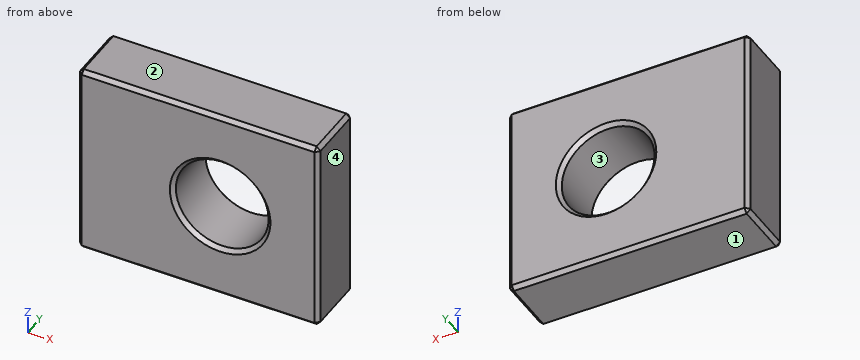
Autodesk Inventor part; units mm, degrees
ref_plane "YZ Plane" through (0, 0, 0) normal (1, 0, 0) x (0, 1, 0)
ref_plane "XZ Plane" through (0, 0, 0) normal (0, 1, 0) x (-1, 0, 0)
ref_plane "XY Plane" through (0, 0, 0) normal (0, 0, 1) x (1, 0, 0)
sketch "Sketch1" plane through (0, 0, 0) normal (0, 1, 0) x (-1, 0, 0)
  line L0 (0, 0) -> (-15.85, 0) construction
  line L1 (-15.85, 0) -> (-15.85, -13) construction
  line L2 (-15.85, -13) -> (0, -13) construction
  line L3 (0, -13) -> (0, 0) construction
  line L4 (0, 0) -> (-9.35, 0) construction
  line L5 (-9.35, 0) -> (-9.35, -6.5) construction
  line L6 (-9.35, -6.5) -> (0, -6.5) construction
  line L7 (0, -6.5) -> (0, 0) construction
  circle A0 centre (-9.35, -6.5) radius 3
  line L8 (0, 0) -> (-0.15, 0) construction
  line L9 (-0.15, 0) -> (-0.15, -0.15) construction
  line L10 (-0.15, -0.15) -> (0, -0.15) construction
  line L11 (0, -0.15) -> (0, 0) construction
  line L12 (-15.85, -13) -> (-15.7, -13) construction
  line L13 (-15.7, -13) -> (-15.7, -12.85) construction
  line L14 (-15.7, -12.85) -> (-15.85, -12.85) construction
  line L15 (-15.85, -12.85) -> (-15.85, -13) construction
  line L16 (-0.15, -0.15) -> (-15.7, -0.15)
  line L17 (-15.7, -0.15) -> (-15.7, -12.85)
  line L18 (-15.7, -12.85) -> (-0.15, -12.85)
  line L19 (-0.15, -12.85) -> (-0.15, -0.15)
  dimension "d0" = 15.85
  dimension "d1" = 13
  dimension "d2" = 9.35
  dimension "d3" = 6.5
  dimension "d4" = 6
extrude "Extrusion1" add sketch "Sketch1" along normal blind 4
chamfer "Chamfer1" distance 0.25 angle 45 14 edges at (0.15, 4, -6.5) (7.925, 4, -12.85) (15.7, 4, -6.5) (7.925, 4, -0.15) (0.15, 2, -0.15) (15.7, 2, -0.15) (15.7, 2, -12.85) (0.15, 2, -12.85) (0.15, 0, -6.5) (7.925, 0, -12.85) (12.35, 4, -6.5) (12.35, 0, -6.5) (15.7, 0, -6.5) (7.925, 0, -0.15)
properties part number "Calza para ventilador"
Geometry check sheet. Reference: the model listing, model coordinates, mm. Face numbers are marked on the shaded views. Give positions to 0.01 mm unless a question says otherwise; leave off trailing zeros. Order: outer loops, then holes, each group sorted by start corner. A loop starts at its lowest first (then second) coordinate and runs counter-clockwise, first axis right, second up.
1. Section check B-B, the plane z = -6.5. Enter the section's corners in (x, y).
2. Thickness scan on L1, parallel to Z at x = 9.35, y = 2.85; L2, parallel to X at y = 1.4, z = -5; L3, parallel to X at y = 1.05, z = -4.5. Record the ranges inside material, lowest first.
3. Section check C-C, the plane y = 2.05. Enter the section's corners in (x, z), and give its area (3 significant figures).
4. Release check for a two-part mould opening along Z. For the marked faces 1, 2, 3 and 4 record: pulls with the +Z half, pulls with the -Z half, needs draft (parallel to the pull), parting line crosses it, or undercut.
5. Gauge pin test, flat end, axial feed: pin 1 Ø5 at (x, z) = (11.5, -2.5) entering from -Y. Record the tip position at first contact, or that the pin passes through.
6. Section check A-A, the plane x = 9.35. Enter the section's corners in (y, z), and give its area (4 significant figures).
Values follow:
1. outline: (0.15, 0.25) - (0.4, 0) - (6.1, 0) - (6.35, 0.25) - (6.35, 3.75) - (6.1, 4) - (0.4, 4) - (0.15, 3.75) - close; (12.35, 0.25) - (12.6, 0) - (15.45, 0) - (15.7, 0.25) - (15.7, 3.75) - (15.45, 4) - (12.6, 4) - (12.35, 3.75) - close
2. L1: z = -12.85 to -9.5, -3.5 to -0.15
2. L2: x = 0.15 to 6.75, 11.95 to 15.7
2. L3: x = 0.15 to 7.11, 11.59 to 15.7
3. outline: (0.15, -12.6) - (0.4, -12.85) - (15.45, -12.85) - (15.7, -12.6) - (15.7, -0.4) - (15.45, -0.15) - (0.4, -0.15) - (0.15, -0.4) - close; hole circle Ø6 at (9.35, -6.5)
3. area: 169 mm2
4. face 1: pulls with the -Z half
4. face 2: pulls with the +Z half
4. face 3: undercut
4. face 4: needs draft
5. pin 1: stops at y = 0
6. outline: (0, -12.6) - (0.25, -12.85) - (3.75, -12.85) - (4, -12.6) - (4, -9.75) - (3.75, -9.5) - (0.25, -9.5) - (0, -9.75) - close; (0, -3.25) - (0.25, -3.5) - (3.75, -3.5) - (4, -3.25) - (4, -0.4) - (3.75, -0.15) - (0.25, -0.15) - (0, -0.4) - close
6. area: 26.55 mm2
